Geometry: final body of the model. Coordinates: model frame, mm. Give positions to 0.01 mm unless a question says otherwise; leave off trailing zeros. Loops run counter-clockwise (first coordinate to the right, second up) from the corner with the lowest first, then second, coordinate; pieces in that order, holes last. Notation, with made-up numbers: M 19,36 L 72,36 A26 ccw 72,71 Z; hole C 54.5,-9 d2. An arc over 180 degrees is marked long. One line per question, with ' | ' between items. Start each with the question number.
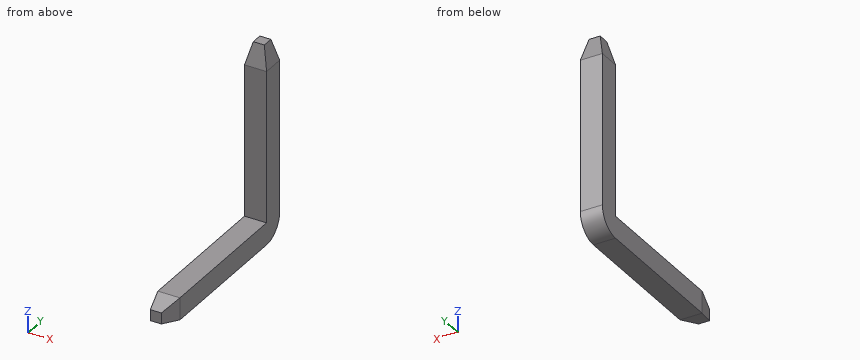
from build123d import *

# Parameters (mm, degrees)
SKETCH_1_W      = 6.9
SKETCH_1_H      = 0.8
EXTRUDE_1_DEPTH = 0.8
SKETCH_2_W      = 0.8
SKETCH_2_H      = 0.8
EXTRUDE_2_DEPTH = 6.3
CHAMFER_1_SIZE  = 0.2
CHAMFER_1_SIZE2 = 0.8
CHAMFER_2_SIZE  = 0.2
CHAMFER_2_SIZE2 = 0.8
FILLET_1_R      = 0.8


with BuildPart() as part:
    # Эскиз1 → Бобышка-Вытянуть1 (new body)
    with BuildSketch(Plane(origin=(-0.4, 0, 0), x_dir=(0, -1, 0), z_dir=(-1, 0, 0))):
        with Locations((-0.4, -3.55)):
            Rectangle(SKETCH_1_W, SKETCH_1_H)
    extrude(amount=-EXTRUDE_1_DEPTH)

    # Эскиз2 → Бобышка-Вытянуть2 (add)
    with BuildSketch(Plane.XY.offset(-3.15)):
        with Locations((0, 3.45)):
            Rectangle(SKETCH_2_W, SKETCH_2_H)
    extrude(amount=EXTRUDE_2_DEPTH)

    # Фаска1
    chamfer_1_edges = [part.edges().sort_by_distance(p)[0] for p in [
        (0, -3.05, -3.15),
        (0.4, -3.05, -3.55),
        (-0.4, -3.05, -3.55),
        (0, -3.05, -3.95),
    ]]
    chamfer_1_side = [part.faces().sort_by_distance(p)[0] for p in [
        (0, -3.05, -3.55),
    ]]
    chamfer(chamfer_1_edges, length=CHAMFER_1_SIZE, length2=CHAMFER_1_SIZE2, reference=chamfer_1_side[0])

    # Фаска2
    chamfer_2_edges = [part.edges().sort_by_distance(p)[0] for p in [
        (0, 3.85, 3.15),
        (0.4, 3.45, 3.15),
        (-0.4, 3.45, 3.15),
        (0, 3.05, 3.15),
    ]]
    chamfer_2_side = [part.faces().sort_by_distance(p)[0] for p in [
        (0, 3.45, 3.15),
    ]]
    chamfer(chamfer_2_edges, length=CHAMFER_2_SIZE, length2=CHAMFER_2_SIZE2, reference=chamfer_2_side[0])

    # Скругление1
    fillet_1_edges = [part.edges().sort_by_distance(p)[0] for p in [
        (0, 3.85, -3.95),
    ]]
    fillet(fillet_1_edges, radius=FILLET_1_R)


solid = part.part
Q1. Section A-A, the plane x = 0.1. Output: boundary loops of the cut face in (y, z), plus the area to 3 significant figures.
Q2. Section D-D, the plane z = -1.25. Output: boundary loops of the cut face in (x, y), plus the area to 3 significant figures.
Q3. Contact query for a flat-ended pin moving along its axis: pin 1 (4 mm diameter, centred on y = -0.5, z = -2.5, fed in from +X). Output: stop coordinate, or through.
Q4. Section C-C, the plane y = -1. Output: boundary loops of the cut face in (x, z), plus the area to 3 significant figures.
Q5. Material intervals for L1, parallel to Z at x = -0.1, y = 1; L2, parallel to Y at x = 0.3, z = 0.75, sorted ascending.
Q6. Section B-B, the plane z = -3.25. Output: boundary loops of the cut face in (x, y), plus the area to 3 significant figures.
Model answer:
1) outline: M -3.05,-3.75 L -2.25,-3.95 L 3.05,-3.95 A0.8 ccw 3.85,-3.15 L 3.85,2.35 L 3.65,3.15 L 3.25,3.15 L 3.05,2.35 L 3.05,-3.15 L -2.25,-3.15 L -3.05,-3.35 Z | area: 10.1 mm^2
2) outline: M -0.4,3.05 L 0.4,3.05 L 0.4,3.85 L -0.4,3.85 Z | area: 0.640 mm^2
3) pin 1: stops at x = 0.4
4) outline: M -0.4,-3.95 L 0.4,-3.95 L 0.4,-3.15 L -0.4,-3.15 Z | area: 0.640 mm^2
5) L1: z = -3.95 to -3.15 | L2: y = 3.05 to 3.85
6) outline: M -0.4,-2.25 L -0.3,-2.65 L 0.3,-2.65 L 0.4,-2.25 L 0.4,3.84 L -0.4,3.84 Z | area: 5.15 mm^2
